Verification items for this drawing (mm, ordinates from the low corner). Coordinates: 2 decimals unless noted, no trailing zeros. Order: outer loops, then holes, each group sorted by start corner. A loop starts at its lowest first (then second) coordinate and runs counter-clockwise, first axis right, second up. Notation, with made-up numbers: M 41,74 L 47,74 A30 cw 47,108 Z; hole C -5.5,78 d5. An arc over 180 degrees is marked long. Use CSV: the item, a comma, the result in double quotes. Start each with the question number.
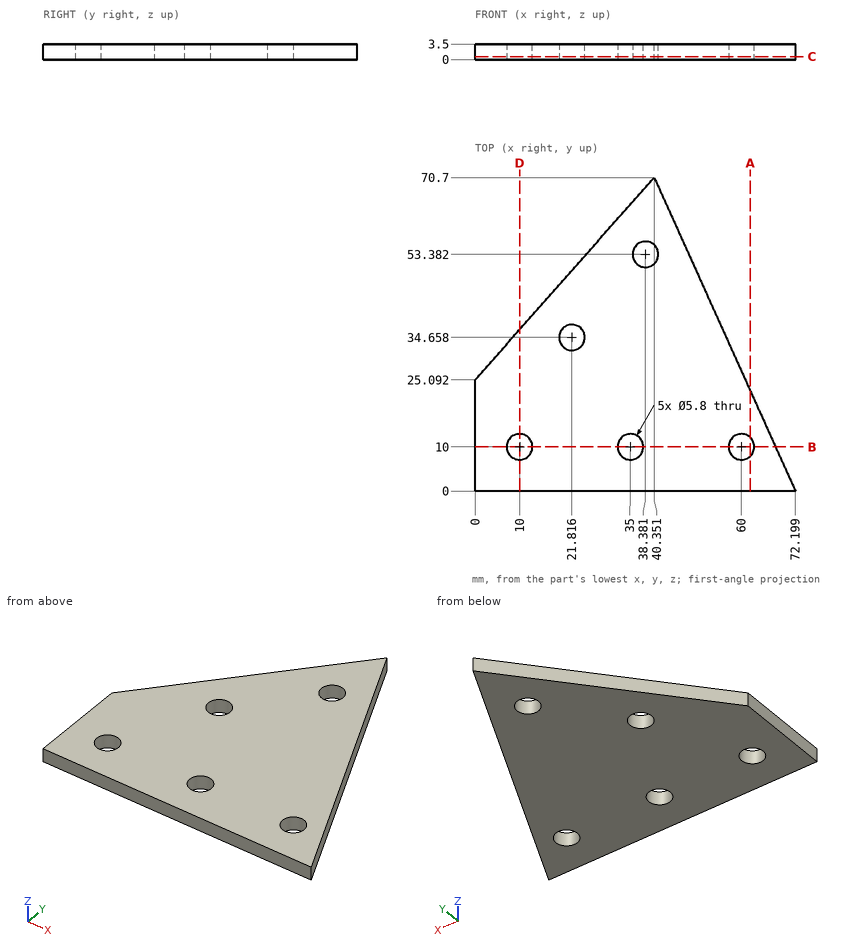
1) Section check A-A on x = 62. Record the boundary of the cut face in (y, z).
2) Section check B-B on y = 10. Record the boundary of the cut face in (x, z) (1 decimal).
3) Gauge pin test, flat ends, axial feed: P1, Ø8, axis at x = 11.5, y = 8, coming from the -Z side; P2, Ø3.5, axis at x = 35, y = 10, coming from the -Z side. Record the tip position at first contact, or that the pin passes through.
4) Material ranges on line 1 along Y through (x, z) = (60, 1.7) (1 decimal); line 2 along Y through (x, z) = (61, 3.3) (1 decimal); line 3 along X through (y, z) = (12, 0.55) (1 decimal), recorded low to high.
5) Section check D-D on x = 10. Record the boundary of the cut face in (y, z) (1 decimal).
6) Section check C-C on z = 0.65. Record the boundary of the cut face in (x, y), then the cut area to 3 significant figures.
Results are:
1,outline,"M 0,0 L 7.9,0 L 7.9,3.5 L 0,3.5 Z; M 12.1,0 L 22.64,0 L 22.64,3.5 L 12.1,3.5 Z"
2,outline,"M 0,0 L 7.1,0 L 7.1,3.5 L 0,3.5 Z; M 12.9,0 L 32.1,0 L 32.1,3.5 L 12.9,3.5 Z; M 37.9,0 L 57.1,0 L 57.1,3.5 L 37.9,3.5 Z; M 62.9,0 L 67.7,0 L 67.7,3.5 L 62.9,3.5 Z"
3,P1,"stops at z = 0"
3,P2,"passes through"
4,line 1,"y = 0 to 7.1, 12.9 to 27.1"
4,line 2,"y = 0 to 7.3, 12.7 to 24.9"
4,line 3,"x = 0 to 7.9, 12.1 to 32.9, 37.1 to 57.9, 62.1 to 66.8"
5,outline,"M 0,0 L 7.1,0 L 7.1,3.5 L 0,3.5 Z; M 12.9,0 L 36.4,0 L 36.4,3.5 L 12.9,3.5 Z"
6,outline,"M 0,0 L 72.2,0 L 40.35,70.7 L 0,25.09 Z; hole C 10,10 d5.8; hole C 21.82,34.66 d5.8; hole C 35,10 d5.8; hole C 38.38,53.38 d5.8; hole C 60,10 d5.8"
6,area,"2,930 mm²"
